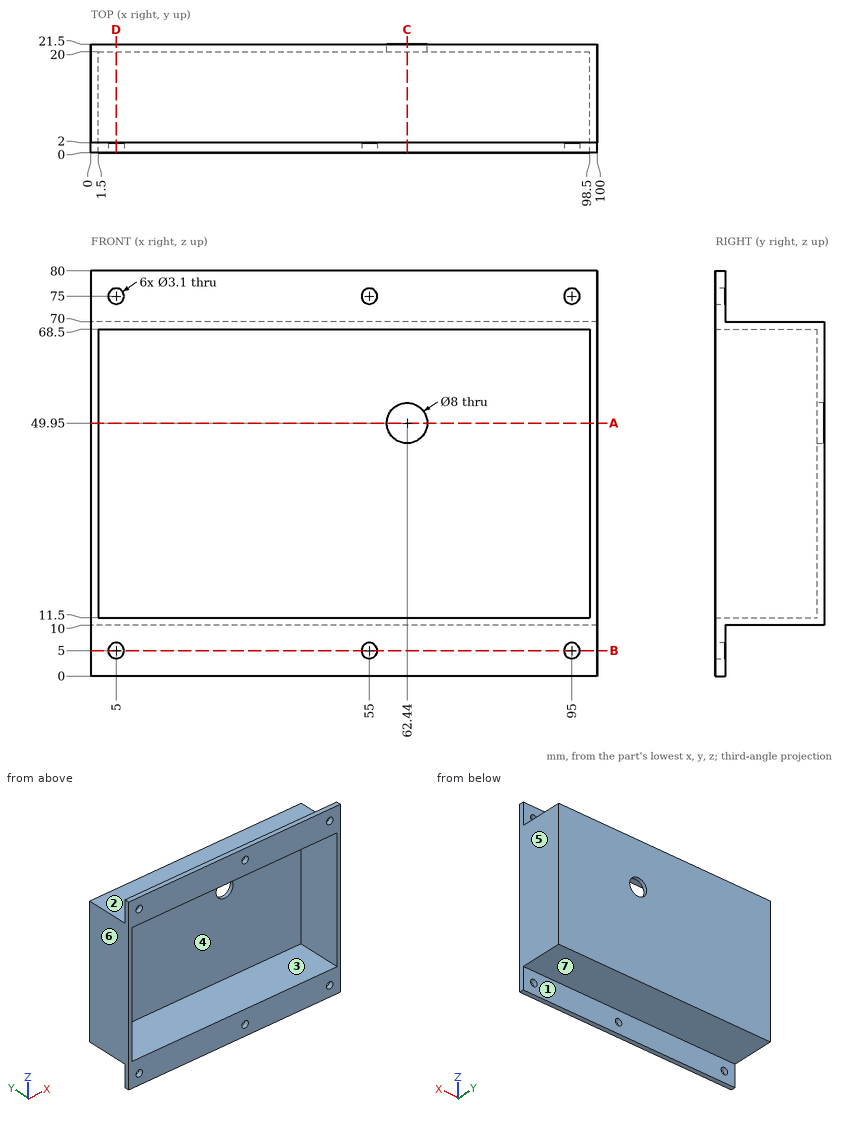
Job drawing, mm, ordinate dimensions from the low corner. One solid piece. A direction names the side the tool comes from. Give positions to 0.01 mm unless a question says otherwise; leave off trailing zeros. Loops run counter-clockwise (first coordinate to the right, second up) from the corner with the lowest first, then second, coordinate; pieces in that order, holes last. Notation, with made-up numbers: M 8,-4.75 L 14,-4.75 A37 ccw 14,31.25 Z; hole C 17.5,26.25 d5. An arc over 180 degrees is marked long. Use one line per item in the form item = value.
Item 1: Which spindle directions (+Z, -Z, +X, -X, +Y, -Y) get a long thin tool onto all of the face, cutting with end or side? Do the marked faces 1, 2 and 3. Say none if no direction does.
Filled in:
face_1 = -Z, +X, -X, +Y
face_2 = +Z, +X, -X, +Y
face_3 = -Y
Item 2: Two-plate mould, pull along X, no slides. Class the marked faces 4, 5, 6 and 7: released by +X, released by -X, zero draft, split by the parting line, or undercut.
Filled in:
face_4 = undercut
face_5 = released by +X
face_6 = released by -X
face_7 = zero draft
Item 3: Flat gauge pins, fed straight in: pin 1 Ø10 at (x, z) = (29.5, 63) entering from -Y; pin 2 Ø4 at (x, z) = (95, 5) entering from +Y; pin 3 Ø2.5 at (x, z) = (95, 75) entering from +Y (1 decimal); pin 4 Ø10 at (x, y) = (33.5, 14) entering from -Z. Where does each tip first touch, or does it go through?
Filled in:
pin_1 = 20
pin_2 = 2
pin_3 = through
pin_4 = 10
Item 4: Drill centre lines: L1, parallel to X at y = 1.15, z = 75; L2, parallel to Z at x = 95, y = 1.15; L3, parallel to Z at x = 34.5, y = 9.75. Where is each one in solid material? Low to high.
Filled in:
L1 = 0 to 3.45, 6.55 to 53.45, 56.55 to 93.45, 96.55 to 100
L2 = 0 to 3.45, 6.55 to 11.5, 68.5 to 73.45, 76.55 to 80
L3 = 10 to 11.5, 68.5 to 70
Item 5: Slice it at A-A on z = 49.95. List the corners of the cut face in (x, y), and give its area (3 significant figures).
Filled in:
outline = M 0,0 L 1.5,0 L 1.5,20 L 58.44,20 L 58.44,21.5 L 0,21.5 Z; M 66.44,20 L 98.5,20 L 98.5,0 L 100,0 L 100,21.5 L 66.44,21.5 Z
area = 198 mm^2
Item 6: Slice it at D-D on x = 5. List the corners of the cut face in (y, z).
Filled in:
outline = M 0,0 L 2,0 L 2,3.45 L 0,3.45 Z; M 0,6.55 L 2,6.55 L 2,10 L 21.5,10 L 21.5,70 L 2,70 L 2,73.45 L 0,73.45 L 0,68.5 L 20,68.5 L 20,11.5 L 0,11.5 Z; M 0,76.55 L 2,76.55 L 2,80 L 0,80 Z
Item 7: Slice it at B-B on z = 5. List the corners of the cut face in (x, y).
Filled in:
outline = M 0,0 L 3.45,0 L 3.45,2 L 0,2 Z; M 6.55,0 L 53.45,0 L 53.45,2 L 6.55,2 Z; M 56.55,0 L 93.45,0 L 93.45,2 L 56.55,2 Z; M 96.55,0 L 100,0 L 100,2 L 96.55,2 Z
Item 8: Slice it at C-C on x = 62.44. List the corners of the cut face in (y, z), and give its area (3 significant figures).
Filled in:
outline = M 0,0 L 2,0 L 2,10 L 21.5,10 L 21.5,45.95 L 20,45.95 L 20,11.5 L 0,11.5 Z; M 0,68.5 L 20,68.5 L 20,53.95 L 21.5,53.95 L 21.5,70 L 2,70 L 2,80 L 0,80 Z
area = 178 mm^2
